Autodesk Inventor part; units mm, degrees
ref_plane "YZ Plane" through (0, 0, 0) normal (1, 0, 0) x (0, 1, 0)
ref_plane "XZ Plane" through (0, 0, 0) normal (0, 1, 0) x (-1, 0, 0)
ref_plane "XY Plane" through (0, 0, 0) normal (0, 0, 1) x (1, 0, 0)
sketch "Sketch1" plane through (0, 0, 0) normal (0, 1, 0) x (-1, 0, 0)
  line L0 (0, 0) -> (63.5, 0)
  line L1 (63.5, 0) -> (63.5, 50.8)
  line L2 (63.5, 50.8) -> (0, 50.8)
  line L3 (0, 50.8) -> (0, 0)
  dimension "cameraWidth" = 63.5
  dimension "cameraDepth" = 50.8
extrude "Extrusion1" add sketch "Sketch1" along normal blind 15.875
sketch "Sketch2" plane through (0, 15.875, 0) normal (0, 1, 0) x (1, 0, 0)
  line L0 (0, -50.8) -> (0, 0)
  line L1 (-63.5, -50.8) -> (0, -50.8)
  line L2 (0, -50.8) -> (0, -34.925)
  line L3 (0, -34.925) -> (-63.5, -34.925)
  line L4 (-63.5, -34.925) -> (-63.5, -50.8)
  dimension "d4" = 15.875
extrude "Extrusion2" add sketch "Sketch2" along normal blind 31.75
sketch "Sketch3" plane through (-63.5, 0, 50.8) normal (0, 0, 1) x (1, 0, 0)
  line L0 (0, 0) -> (63.5, 0)
  line L1 (0, 0) -> (0, 47.625)
  circle A0 centre (31.75, 31.75) radius 12.7
  dimension "d7" = 31.75
  dimension "cameraLensHeight" = 31.75
  dimension "d9" = 25.4
extrude "Extrusion3" cut sketch "Sketch3" against normal blind 2.54
sketch "Sketch4" plane through (-63.5, 0, 50.8) normal (0, 0, 1) x (1, 0, 0)
  circle A0 centre (31.75, 31.75) radius 12.7
  line L0 (0, 0) -> (63.5, 0)
  line L1 (63.5, 0) -> (63.5, 47.625)
  line L2 (0, 47.625) -> (63.5, 47.625)
  line L3 (0, 0) -> (0, 47.625)
  line L4 (0, 31.75) -> (63.5, 31.75)
  line L5 (31.75, 47.625) -> (31.75, 0)
  dimension "d12" = 31.75
sketch "Sketch5" plane through (0, 0, 0) normal (0, -1, 0) x (1, 0, 0)
  line L0 (0, 0) -> (-63.5, 0)
  line L1 (0, 50.8) -> (0, 0)
  line L2 (-63.5, 50.8) -> (0, 50.8)
  line L3 (-63.5, 0) -> (-63.5, 50.8)
  line L4 (-63.5, 22.225) -> (0, 22.225)
  line L5 (-31.75, 50.8) -> (-31.75, 0)
  circle A0 centre (-31.75, 22.225) radius 7.8401
  dimension "cameraMountingHoleDistanceFromFront" = 28.575
hole "Hole1" at (-31.75, 0, 22.225) direction (0, 1, 0) diameter 4.9784 depth 8.43
equation "\"d7\" = 0.5 * cameraWidth"
equation "\"d12\" = cameraLensHeight"
properties part number "camera"
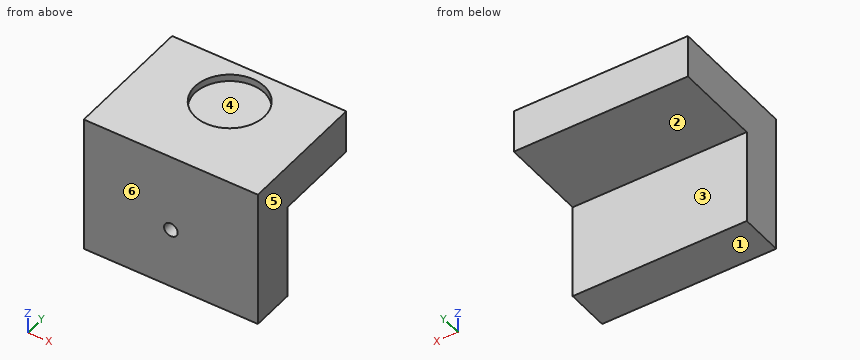
Verification items for the finished model (mm, model axes). Face numbers are marked on the shaded views. A direction names the side the tool comes from. Give positions to 0.01 mm unless a question says otherwise; leave off trailing zeros. Write each loop counter-clockwise with the first axis right and the second up, starting at its lowest first coordinate (ties: lowest second). Pieces come first, ordered by that corner, then holes. Notation, with made-up numbers: M 75.25,25 L 93.25,25 A21 cw 93.25,48 Z; hole C -0.5,-15.5 d11. An arc over 180 degrees is marked long. Use CSV: the item, a comma, the result in double quotes.
1) Go/stop test with flat-tipped pins: pin 1 Ø1.5 at (x, z) = (-31, 22) entering from +Y (3 decimals); pin 2 Ø1 at (x, z) = (-35.5, 33) entering from -Y; pin 3 Ø2.5 at (x, z) = (-31.5, 22) entering from -Y; pin 4 Ø5 at (x, y) = (-46.5, 33.5) entering from -Z (3 decimals). Record where each tip stops, or that it passes through.
Final values:
pin 1,"y = 15.875"
pin 2,"y = 0"
pin 3,"y = 8.43"
pin 4,"z = 34.925"
2) Cross-section at D-D (z = 29.5). Enter the section's corners in (x, y) (3 decimals).
Final values:
outline,"M -63.5,0 L 0,0 L 0,15.875 L -63.5,15.875 Z"
3) Cross-section at B-B (x = -31.75). Enter the section's corners in (y, z) (3 decimals).
Final values:
outline,"M 0,0 L 15.875,0 L 15.875,34.925 L 47.625,34.925 L 47.625,50.8 L 44.45,50.8 L 44.45,48.26 L 19.05,48.26 L 19.05,50.8 L 0,50.8 L 0,24.714 L 8.43,24.714 L 8.43,19.736 L 0,19.736 Z"
4) Cross-section at A-A (y = 31.75). Enter the section's corners in (x, z) (3 decimals), plus the area to 3 significant figures.
Final values:
outline,"M -63.5,34.925 L 0,34.925 L 0,50.8 L -19.05,50.8 L -19.05,48.26 L -44.45,48.26 L -44.45,50.8 L -63.5,50.8 Z"
area,"944 mm²"
5) Release check for a two-part mould opening along Y. For the marked faces 3, 4, 5 and 6 record: released by +Y, released by -Y, zero draft, split by the parting line, or undercut.
Final values:
face 3,"released by +Y"
face 4,"undercut"
face 5,"zero draft"
face 6,"released by -Y"
6) Cross-section at C-C (x = -13.5). Enter the section's corners in (y, z) (3 decimals), plus the area to 3 significant figures.
Final values:
outline,"M 0,0 L 15.875,0 L 15.875,34.925 L 47.625,34.925 L 47.625,50.8 L 0,50.8 Z"
area,"1,310 mm²"
7) Material ranges on line 1 along Y through (x, z) = (-31.75, 49.05) (3 decimals); line 2 along Z through (x, y) = (-31.75, 4.5); line 3 along Z through (x, y) = (-21.5, 33) (3 decimals), recorded low to high.
Final values:
line 1,"0 to 19.05, 44.45 to 47.625"
line 2,"0 to 19.74, 24.71 to 50.8"
line 3,"34.925 to 48.26"
8) Access from +Z, -Z, +X, -X, +Y, -Y to the whole of each face (thin tool, end or side, straight path). Record for the marked faces 1 and 2.
Final values:
face 1,"-Z, +X, -X, +Y, -Y"
face 2,"-Z, +X, -X, +Y"
